The listing builds one solid part. Answer for the finished solid, in the listing's coordinates (mm). A direction names the side the tool comes from. Round coordinates to 2 decimals unless told otherwise and drop trailing zeros. Order: outer loops, then holes, each group sorted by start corner. A loop starts at its lowest first (then second) coordinate and runs counter-clockwise, first axis right, second up. Notation, with made-up numbers: (28, 57) -> (71, 57) arc R16 cw to (71, 65) -> close; hole circle Ø11 at (-1, -16). An arc over 180 degrees is marked (long way). Return JSON: item names as keys, results as strings. Group by question number.
(1) The part is cut by section C-C (x = 9). Determine the outline of the cut face in (y, z), plus the area to 3 significant figures.
(2) Each of these flat-tipped pins is pushed along its axis until it touches: pin 1 (4 mm diameter, centred on x = 66.14, z = 29.4, fed in from +Y); pin 2 (1.8 mm diameter, centred on x = -5.5, z = 23, fed in from -Y); pin 3 (1.8 mm diameter, centred on x = -34, z = -24.5, fed in from -Y). Where does it stop, or does it pass through?
(3) Which of the six approach directions +Z, -Z, +X, -X, +Y, -Y give full straight-line access (tool end or side, diameter ignored) to faces 1 (the face through (13, 0, 33)), 2 (the face through (-17.513, 41, 0)), 3 (the face through (67.737, 19, 0))?
(4) The part is cut by section B-B (y = 18). Determine the outline of the cut face in (x, z).
(5) Consider line 1 (X direction, y = 31, z = -29.5); line 2 (X direction, y = 27.5, z = -15); line 3 (Z direction, x = 60, y = 20). Determine where each line is inside the solid, lowest interval first. Write a range as [from, to].
(6) Determine the mould class of faces 4 (the face through (-44.763, 21, 0)), 5 (the face through (69.88, 21.2, -33.1)), 6 (the face through (55, 39, -24)) for opening direction Z: +Z half, -Z half, draft (parallel to the pull), parting line (faces both ways), or undercut.
(7) The part is cut by section A-A (z = 17.5). Determine the outline of the cut face in (x, y), plus the area to 3 significant figures.
from build123d import *

# Parameters (mm, degrees)
SKETCH_3_W          = 109.5
SKETCH_3_H          = 62
EXTRUDE_2_DEPTH     = 40
SKETCH_5_R          = 1.6
EXTRUDE_2_2_DEPTH   = 40
SKETCH_7_R          = 1.6
EXTRUDE_3_DEPTH     = 3
CHAMFER_1_SIZE      = 1.5
SKETCH_9_R          = 3
SKETCH_9_R_2        = 0.75
EXTRUDE_4_DEPTH     = 3
SKETCH_10_R         = 1.6
SKETCH_10_W         = 20.5
SKETCH_10_H         = 40.5
CUT_EXTRUDE_1_DEPTH = 4
CHAMFER_2_SIZE      = 1.5
FILLET_2_R          = 1.5
FILLET_3_R          = 1.5
SKETCH_12_R         = 3
SKETCH_12_R_2       = 1.6
EXTRUDE_5_DEPTH     = 2


with BuildPart() as part:
    # Эскиз3 → Extrude 2 (new body)
    with BuildSketch(Plane(origin=(0, 0, 0), x_dir=(1, 0, 0), z_dir=(0, 1, 0))):
        with BuildLine():
            Line((-41.762564045, 34), (67.737435955, 34))
            ThreePointArc((67.737435955, 34), (69.858756299, 33.121320344), (70.737435955, 31))
            Line((70.737435955, 31), (70.737435955, -31))
            ThreePointArc((70.737435955, -31), (69.858756299, -33.121320344), (67.737435955, -34))
            Line((67.737435955, -34), (-41.762564045, -34))
            ThreePointArc((-41.762564045, -34), (-43.883884388, -33.121320344), (-44.762564045, -31))
            Line((-44.762564045, -31), (-44.762564045, 31))
            ThreePointArc((-44.762564045, 31), (-43.883884388, 33.121320344), (-41.762564045, 34))
        make_face()
        with Locations((12.987435955, 0)):
            Rectangle(SKETCH_3_W, SKETCH_3_H, mode=Mode.SUBTRACT)
    extrude(amount=EXTRUDE_2_DEPTH)

    # Эскиз5 → Extrude 2 2 (add)
    with BuildSketch(Plane.XZ):
        with BuildLine():
            Line((-43.498616626, 27), (-43.498616626, 32.026898844))
            Line((-43.498616626, 32.026898844), (-37.762564045, 32.026898844))
            Line((-37.762564045, 32.026898844), (-37.762564045, 28.5))
            ThreePointArc((-37.762564045, 28.5), (-38.201903873, 27.439339828), (-39.262564045, 27))
            Line((-39.262564045, 27), (-43.498616626, 27))
        make_face()
        with Locations((-40.162564045, 29.4)):
            Circle(SKETCH_5_R, mode=Mode.SUBTRACT)
        with BuildLine():
            Line((-43.498616626, -32.026898844), (-37.762564045, -32.026898844))
            Line((-37.762564045, -32.026898844), (-37.762564045, -28.5))
            ThreePointArc((-37.762564045, -28.5), (-38.201903873, -27.439339828), (-39.262564045, -27))
            Line((-39.262564045, -27), (-43.498616626, -27))
            Line((-43.498616626, -27), (-43.498616626, -32.026898844))
        make_face()
        with Locations((-40.162564045, -29.4)):
            Circle(SKETCH_5_R, mode=Mode.SUBTRACT)
        with BuildLine():
            Line((69.473488536, -27), (69.473488536, -32.026898844))
            Line((69.473488536, -32.026898844), (63.737435955, -32.026898844))
            Line((63.737435955, -32.026898844), (63.737435955, -28.5))
            ThreePointArc((63.737435955, -28.5), (64.176775783, -27.439339828), (65.237435955, -27))
            Line((65.237435955, -27), (69.473488536, -27))
        make_face()
        with Locations((66.137435955, -29.4)):
            Circle(SKETCH_5_R, mode=Mode.SUBTRACT)
        with BuildLine():
            Line((69.473488536, 32.026898844), (63.737435955, 32.026898844))
            Line((63.737435955, 32.026898844), (63.737435955, 28.5))
            ThreePointArc((63.737435955, 28.5), (64.176775783, 27.439339828), (65.237435955, 27))
            Line((65.237435955, 27), (69.473488536, 27))
            Line((69.473488536, 27), (69.473488536, 32.026898844))
        make_face()
        with Locations((66.137435955, 29.4)):
            Circle(SKETCH_5_R, mode=Mode.SUBTRACT)
    extrude(amount=-EXTRUDE_2_2_DEPTH)

    # Эскиз7 → Бобышка-Вытянуть3 (add)
    with BuildSketch(Plane(origin=(0, 40, 0), x_dir=(1, 0, 0), z_dir=(0, 1, 0))):
        with BuildLine():
            Line((70.737435955, -31), (70.737435955, 31))
            ThreePointArc((70.737435955, 31), (69.858756299, 33.121320344), (67.737435955, 34))
            Line((67.737435955, 34), (-41.762564045, 34))
            ThreePointArc((-41.762564045, 34), (-43.883884388, 33.121320344), (-44.762564045, 31))
            Line((-44.762564045, 31), (-44.762564045, -31))
            ThreePointArc((-44.762564045, -31), (-43.883884388, -33.121320344), (-41.762564045, -34))
            Line((-41.762564045, -34), (67.737435955, -34))
            ThreePointArc((67.737435955, -34), (69.858756299, -33.121320344), (70.737435955, -31))
        make_face()
        with Locations((66.137435955, 29.4)):
            Circle(SKETCH_7_R, mode=Mode.SUBTRACT)
        with Locations((66.137435955, -29.4)):
            Circle(SKETCH_7_R, mode=Mode.SUBTRACT)
        with Locations((-40.162564045, -29.4)):
            Circle(SKETCH_7_R, mode=Mode.SUBTRACT)
        with Locations((-40.162564045, 29.4)):
            Circle(SKETCH_7_R, mode=Mode.SUBTRACT)
    extrude(amount=EXTRUDE_3_DEPTH)

    # Фаска1
    chamfer_1_edges = [part.edges().sort_by_distance(p)[0] for p in [
        (64.537435955, 43, -29.4),
        (64.537435955, 43, 29.4),
        (-41.762564045, 43, 29.4),
        (-41.762564045, 43, -29.4),
    ]]
    chamfer(chamfer_1_edges, length=CHAMFER_1_SIZE)

    # Эскиз9 → Бобышка-Вытянуть4 (add)
    with BuildSketch(Plane.XZ.offset(-40)):
        with Locations((-6.762564044, 22.000000001)):
            Circle(SKETCH_9_R)
        with Locations((-6.762564044, 22.000000001)):
            Circle(SKETCH_9_R_2, mode=Mode.SUBTRACT)
        with Locations((57.237435954, 22.000000001)):
            Circle(SKETCH_9_R)
        with Locations((57.237435954, 22.000000001)):
            Circle(SKETCH_9_R_2, mode=Mode.SUBTRACT)
        with Locations((57.237435954, -21.999999999)):
            Circle(SKETCH_9_R)
        with Locations((57.237435954, -21.999999999)):
            Circle(SKETCH_9_R_2, mode=Mode.SUBTRACT)
        with Locations((-6.762564044, -21.999999999)):
            Circle(SKETCH_9_R)
        with Locations((-6.762564044, -21.999999999)):
            Circle(SKETCH_9_R_2, mode=Mode.SUBTRACT)
    extrude(amount=EXTRUDE_4_DEPTH)

    # Эскиз10 → Вырез-Вытянуть1 (cut, through all)
    with BuildSketch(Plane.XZ.offset(-40)):
        with Locations((-33.262564045, 24.5)):
            Circle(SKETCH_10_R)
        with Locations((-22.262564045, -24.5)):
            Circle(SKETCH_10_R)
        with Locations((-27.762564045, 0)):
            Rectangle(SKETCH_10_W, SKETCH_10_H)
    extrude(amount=-CUT_EXTRUDE_1_DEPTH, mode=Mode.SUBTRACT)

    # Фаска2
    chamfer_2_edges = [part.edges().sort_by_distance(p)[0] for p in [
        (-34.862564045, 43, 24.5),
        (-23.862564045, 43, -24.5),
    ]]
    chamfer(chamfer_2_edges, length=CHAMFER_2_SIZE)

    # Скругление2
    fillet_2_edges = [part.edges().sort_by_distance(p)[0] for p in [
        (12.987435955, 40, 31),
    ]]
    fillet(fillet_2_edges, radius=FILLET_2_R)

    # Скругление3
    fillet_3_edges = [part.edges().sort_by_distance(p)[0] for p in [
        (67.737435955, 40, 0),
        (-41.762564045, 40, 0),
        (12.987435955, 40, -31),
    ]]
    fillet(fillet_3_edges, radius=FILLET_3_R)

    # Эскиз12 → Бобышка-Вытянуть5 (add)
    with BuildSketch(Plane.XZ.offset(-40)):
        with Locations((-33.262564045, 24.5)):
            Circle(SKETCH_12_R)
        with Locations((-33.262564045, 24.5)):
            Circle(SKETCH_12_R_2, mode=Mode.SUBTRACT)
        with Locations((-22.262564045, -24.5)):
            Circle(SKETCH_12_R)
        with Locations((-22.262564045, -24.5)):
            Circle(SKETCH_12_R_2, mode=Mode.SUBTRACT)
        with Locations((-33.262564045, -24.5)):
            Circle(SKETCH_12_R)
        with Locations((-22.262564045, 24.5)):
            Circle(SKETCH_12_R)
    extrude(amount=EXTRUDE_5_DEPTH)


solid = part.part
Answer below:
{
 "1": {"outline": "(0, -34) -> (43, -34) -> (43, 34) -> (0, 34) -> (0, 31) -> (38.5, 31) arc R1.5 cw to (40, 29.5) -> (40, -29.5) arc R1.5 cw to (38.5, -31) -> (0, -31) -> close", "area": "445 mm²"},
 "2": {"pin 1": "stops at y = 41.9", "pin 2": "stops at y = 37", "pin 3": "stops at y = 38"},
 "3": {"face 1": "+Z, -Z, +X, -X, -Y", "face 2": "+Y, -Y", "face 3": "-Y"},
 "4": {"outline": "(-44.76, -31) arc R3 ccw to (-41.76, -34) -> (67.74, -34) arc R3 ccw to (70.74, -31) -> (70.74, 31) arc R3 ccw to (67.74, 34) -> (-41.76, 34) arc R3 ccw to (-44.76, 31) -> close; hole circle Ø3.2 at (-40.16, -29.4); hole (-41.76, -27) -> (-39.26, -27) arc R1.5 cw to (-37.76, -28.5) -> (-37.76, -31) -> (63.74, -31) -> (63.74, -28.5) arc R1.5 cw to (65.24, -27) -> (67.74, -27) -> (67.74, 27) -> (65.24, 27) arc R1.5 cw to (63.74, 28.5) -> (63.74, 31) -> (-37.76, 31) -> (-37.76, 28.5) arc R1.5 cw to (-39.26, 27) -> (-41.76, 27) -> close; hole circle Ø3.2 at (-40.16, 29.4); hole circle Ø3.2 at (66.14, -29.4); hole circle Ø3.2 at (66.14, 29.4)"},
 "5": {"line 1": "x = [-44.76, -41.76], [-38.57, -37.76], [63.74, 64.54], [67.73, 70.74]", "line 2": "x = [-44.76, -41.76], [67.74, 70.74]", "line 3": "z = [-34, -31], [31, 34]"},
 "6": {"face 4": "draft", "face 5": "-Z half", "face 6": "undercut"},
 "7": {"outline": "(-44.76, 0) -> (-41.76, 0) -> (-41.76, 38.5) arc R1.5 cw to (-40.26, 40) -> (-38.01, 40) -> (-38.01, 43) -> (-44.76, 43) -> close; (-17.51, 40) -> (66.24, 40) arc R1.5 cw to (67.74, 38.5) -> (67.74, 0) -> (70.74, 0) -> (70.74, 43) -> (-17.51, 43) -> close", "area": "526 mm²"}
}
